Geometry check sheet. Reference: the model listing, model coordinates, mm. Face numbers are marked on the shaded views. A direction names the side the tool comes from. Round coordinates to 2 decimals unless told otherwise and drop trailing zeros. Order: outer loops, then holes, each group sorted by start corner. A loop starts at its lowest first (then second) coordinate and runs counter-clockwise, first axis right, second up. Notation, with made-up numbers: (59, 43) - (108, 43) arc R19 ccw to (108, 60) - close; hole circle Ø11 at (52, 72.25). An arc over 180 degrees is marked (long way). One line per question, with ' | ' between items. Start each with the question number.
Q1. Tool access check on the marked faces 1, 2, 3, 4 and 5. Record the directions out of +Z, -Z, +X, -X, +Y, -Y that give a thin tool (end or side, any length) a straight path to the whole face; none if there is none.
Q2. Mould release check, pull along X, two halves, no side actions. Record for the marked faces 6, 7 and 8: +X half, -X half, draft (parallel to the pull), parting line (faces both ways), or undercut.
Q3. Sectioned sample at B-B, the plane x = 3. Enter the section's corners in (y, z).
Q4. Gauge pin test, flat ends, axial feed: P1, Ø5, axis at x = 10, z = 6, coming from the +Y side; P2, Ø2, axis at x = 16, y = 9.5, coming from the -Z side; P3, Ø1.4, axis at x = -3.5, z = 7.5, coming from the +Y side; P4, Ø5.5, axis at y = 7.5, z = 9, coming from the -X side. Record the tip position at first contact, or that the pin passes through.
Q5. Material ranges on line 1 along X through (y, z) = (5, 14); line 2 along X through (y, z) = (5.5, 9.5); line 3 along Y through (x, z) = (18, 3), recorded low to high.
Q6. Sectioned sample at C-C, the plane x = -0.5. Enter the section's corners in (y, z), then the cut area to 3 significant figures.
Q7. Sectioned sample at A-A, the plane z = -4. Enter the section's corners in (x, y), then the cut area to 3 significant figures.
Q8. Sectioned sample at D-D, the plane y = -0.5. Enter the section's corners in (x, z), then the cut area to 3 significant figures.
```python
from build123d import *

# Parameters (mm, degrees)
SKETCH1_W             = 25
SKETCH1_H             = 11
EXTRUDE1_DEPTH        = 16
SKETCH2_W             = 30
SKETCH2_H             = 14
EXTRUDE2_DEPTH        = 2.3
CHAMFER1_SIZE         = 1.8
CHAMFER1_SIZE2        = 2
CHAMFER1_PART_2_SIZE  = 1.8
CHAMFER1_PART_2_SIZE2 = 2
CHAMFER2_SIZE         = 1.8
CHAMFER2_SIZE2        = 2.5
CHAMFER2_PART_2_SIZE  = 1.8
CHAMFER2_PART_2_SIZE2 = 2.5
EXTRUDE3_DEPTH        = 3.75
EXTRUDE4_DEPTH        = 4.35
EXTRUDE4_DEPTH_BACK   = 4.35
FILLET1_R             = 0.5
SKETCH7_W             = 25
SKETCH7_H             = 2.5
CUT_EXTRUDE2_DEPTH    = 0.44
SKETCH8_R             = 0.9
EXTRUDE5_DEPTH        = 0.8
LPATTERN1_COUNT       = 2
LPATTERN1_PITCH       = 13
LPATTERN2_COUNT       = 2
LPATTERN2_PITCH       = 21.5


with BuildPart() as part:
    # Sketch1 → Extrude1 (new body)
    with BuildSketch(Plane.XY):
        with Locations((12.5, 5.5)):
            Rectangle(SKETCH1_W, SKETCH1_H)
    extrude(amount=EXTRUDE1_DEPTH)

    # Sketch2 → Extrude2 (add)
    with BuildSketch(Plane.XY.offset(16)):
        with Locations((12.5, 5.5)):
            Rectangle(SKETCH2_W, SKETCH2_H)
    extrude(amount=EXTRUDE2_DEPTH)

    # Chamfer1
    chamfer1_edges = [part.edges().sort_by_distance(p)[0] for p in [
        (12.5, -1.5, 18.3),
    ]]
    chamfer1_side = [part.faces().sort_by_distance(p)[0] for p in [
        (12.5, -1.5, 17.15),
    ]]
    chamfer(chamfer1_edges, length=CHAMFER1_SIZE, length2=CHAMFER1_SIZE2, reference=chamfer1_side[0])

    # Chamfer1 part 2
    chamfer1_part_2_edges = [part.edges().sort_by_distance(p)[0] for p in [
        (12.5, 12.5, 18.3),
    ]]
    chamfer1_part_2_side = [part.faces().sort_by_distance(p)[0] for p in [
        (12.5, 12.5, 17.15),
    ]]
    chamfer(chamfer1_part_2_edges, length=CHAMFER1_PART_2_SIZE, length2=CHAMFER1_PART_2_SIZE2, reference=chamfer1_part_2_side[0])

    # Chamfer2
    chamfer2_edges = [part.edges().sort_by_distance(p)[0] for p in [
        (27.5, 5.5, 18.3),
    ]]
    chamfer2_side = [part.faces().sort_by_distance(p)[0] for p in [
        (27.5, 5.5, 17.080769231),
    ]]
    chamfer(chamfer2_edges, length=CHAMFER2_SIZE, length2=CHAMFER2_SIZE2, reference=chamfer2_side[0])

    # Chamfer2 part 2
    chamfer2_part_2_edges = [part.edges().sort_by_distance(p)[0] for p in [
        (-2.5, 5.5, 18.3),
    ]]
    chamfer2_part_2_side = [part.faces().sort_by_distance(p)[0] for p in [
        (-2.5, 5.5, 17.080769231),
    ]]
    chamfer(chamfer2_part_2_edges, length=CHAMFER2_PART_2_SIZE, length2=CHAMFER2_PART_2_SIZE2, reference=chamfer2_part_2_side[0])

    # Sketch4 → Extrude3 (add, symmetric)
    with BuildSketch(Plane(origin=(0, 5.5, 0), x_dir=(-1, 0, 0), z_dir=(0, 1, 0))):
        Polygon((0, 0.892834517), (4.5, 11), (4.264164993, 15.5), (3.265535458, 15.447664044), (3.488805714, 11.187413783), (0, 3.351427853), align=None)
    extrude3 = extrude(amount=EXTRUDE3_DEPTH, both=True)

    # Mirror1: Extrude3 across plane
    add(extrude3.mirror(Plane(origin=(12.5, 0, 0), x_dir=(0, 0, 1), z_dir=(1, 0, 0))))

    # Sketch6 → Extrude4 (add, two sides)
    with BuildSketch(Plane(origin=(0, 5.5, 0), x_dir=(-1, 0, 0), z_dir=(0, 1, 0))) as extrude4_sk:
        with BuildLine():
            Line((-1.2, 18.3), (-1.710738672, 20.15))
            Line((-1.710738672, 20.15), (-12.18088144, 20.15))
            Line((-12.18088144, 20.15), (-20.793792675, 24.7))
            ThreePointArc((-20.793792675, 24.7), (-23.177832074, 21.913793041), (-23.8, 18.3))
            Line((-23.8, 18.3), (-1.2, 18.3))
        make_face()
    extrude(amount=EXTRUDE4_DEPTH)
    extrude(extrude4_sk.sketch, amount=-EXTRUDE4_DEPTH_BACK)

    # Fillet1
    fillet1_edges = [part.edges().sort_by_distance(p)[0] for p in [
        (1.455369336, 1.15, 19.225),
        (1.710738672, 5.5, 20.15),
        (6.945810056, 1.15, 20.15),
        (12.18088144, 5.5, 20.15),
        (16.487337058, 1.15, 22.425),
        (20.793792675, 5.5, 24.7),
        (23.177832074, 1.15, 21.913793041),
        (1.455369336, 9.85, 19.225),
        (6.945810056, 9.85, 20.15),
        (16.487337058, 9.85, 22.425),
        (23.177832074, 9.85, 21.913793041),
    ]]
    fillet(fillet1_edges, radius=FILLET1_R)

    # Sketch7 → Cut-Extrude2 (cut)
    with BuildSketch(Plane.XZ):
        with Locations((12.5, 6.25)):
            Rectangle(SKETCH7_W, SKETCH7_H)
    extrude(amount=-CUT_EXTRUDE2_DEPTH, mode=Mode.SUBTRACT)

    # Sketch8 → Extrude5 (add)
    with BuildSketch(Plane(origin=(1.985092303, 0.243738687, 0), x_dir=(0, 0, -1), z_dir=(0.992546152, 0.121869343, 0))):
        Polygon((8.3, 1.992800038), (9.3, 2.992800038), (9.3, 7.242800038), (8.3, 8.242800038), (0.5, 8.242800038), (0, 7.742800038), (0, 2.492800038), (0.5, 1.992800038), align=None)
        with Locations((6.3, 5.117800038)):
            Circle(SKETCH8_R, mode=Mode.SUBTRACT)
    extrude5 = extrude(amount=EXTRUDE5_DEPTH)

    # LPattern1: Extrude5 ×2
    with Locations(*[(i * LPATTERN1_PITCH, 0, 0) for i in range(1, LPATTERN1_COUNT)]):
        add(extrude5)

    # LPattern2: Extrude5 ×2
    with Locations(*[(i * LPATTERN2_PITCH, 0, 0) for i in range(1, LPATTERN2_COUNT)]):
        add(extrude5)


solid = part.part
```
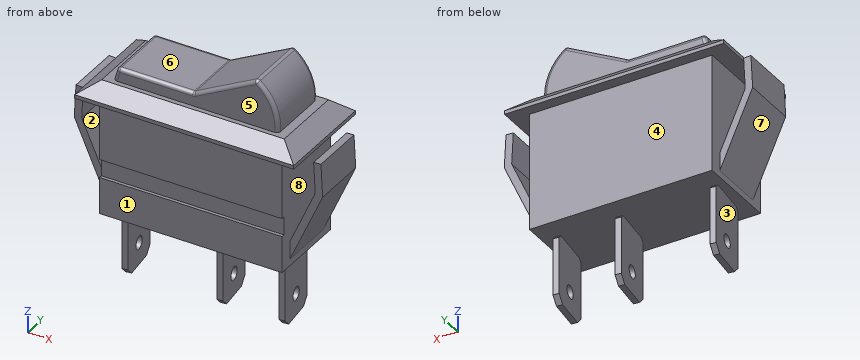
Determined:
1) face 1: -Z, +X, -X, -Y | face 2: +Y, -Y | face 3: -Z, -X, -Y | face 4: -Z, +X, -X, +Y | face 5: +Z, +X, -X, -Y
2) face 6: draft | face 7: -X half | face 8: undercut
3) outline: (-1.5, 16) - (0, 16) - (0, 7.5) - (0.44, 7.5) - (0.44, 5) - (0, 5) - (0, 0) - (11, 0) - (11, 16) - (12.5, 16) - (12.5, 16.5) - (10.5, 18.3) - (9.85, 18.3) - (9.85, 19.65) arc R0.5 ccw to (9.35, 20.15) - (1.65, 20.15) arc R0.5 ccw to (1.15, 19.65) - (1.15, 18.3) - (0.5, 18.3) - (-1.5, 16.5) - close
4) P1: stops at y = 11 | P2: stops at z = 0 | P3: stops at y = 9.25 | P4: stops at x = -4.5
5) line 1: x = -4.34 to -3.34, 0 to 25, 28.34 to 29.34 | line 2: x = -3.83 to -2.74, 0 to 25, 27.74 to 28.83 | line 3: y = 0 to 11
6) outline: (-1.5, 16) - (12.5, 16) - (12.5, 16.5) - (10.9, 17.94) - (0.1, 17.94) - (-1.5, 16.5) - close; (1.75, 2.02) - (9.25, 2.02) - (9.25, 4.47) - (1.75, 4.47) - close | area: 43.3 mm2
7) outline: (0.98, 8.43) - (1.74, 2.22) - (2.54, 2.32) - (1.77, 8.52) - close; (13.98, 8.43) - (14.74, 2.22) - (15.54, 2.32) - (14.77, 8.52) - close; (22.48, 8.43) - (23.24, 2.22) - (24.04, 2.32) - (23.27, 8.52) - close | area: 15.0 mm2
8) outline: (-2.5, 16) - (27.5, 16) - (27.5, 16.5) - (26.25, 17.4) - (-1.25, 17.4) - (-2.5, 16.5) - close | area: 40.9 mm2
